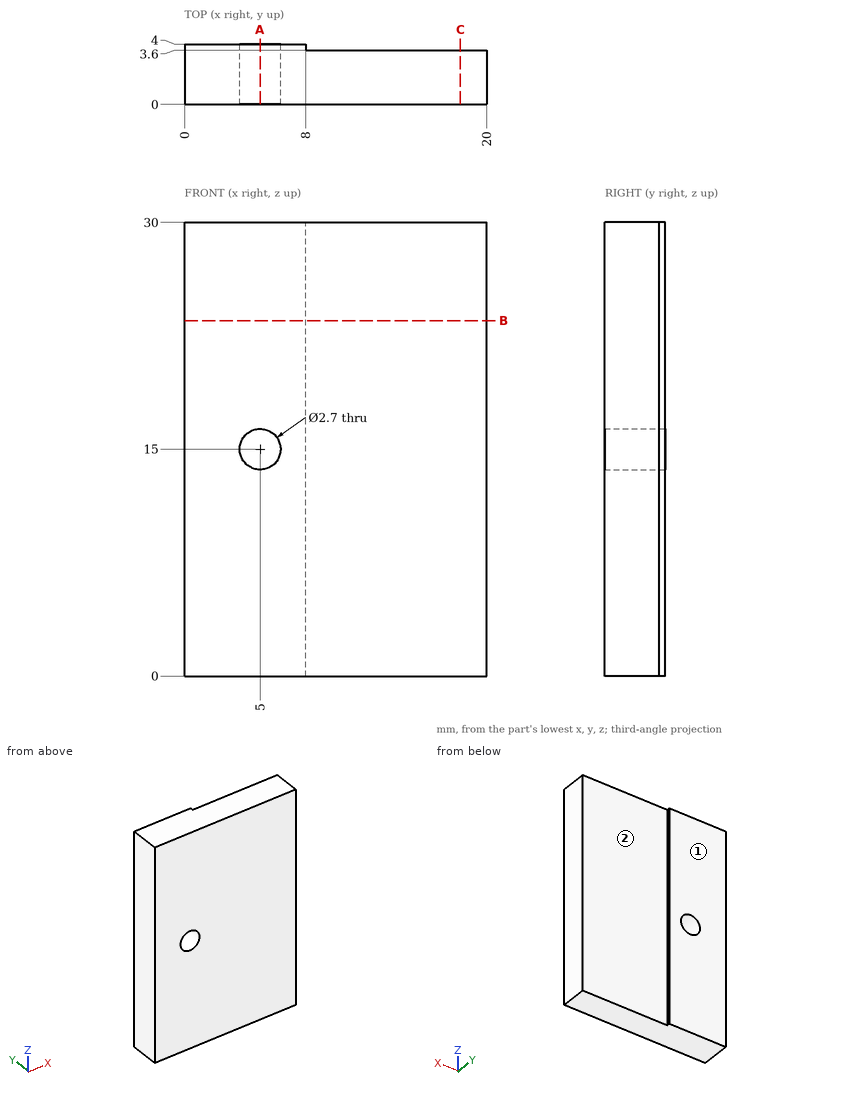
Here's the drawing with two shaded views (mm, measured from the low corner). I have some questions. A direction names the side the tool comes from. Coordinates: 2 decimals unless noted, no trailing zeros. Loops run counter-clockwise (first coordinate to the right, second up) from the corner with the lowest first, then second, coordinate; pieces in that order, holes last. Notation, with made-up numbers: M 76,41.5 L 80,41.5 A30 ccw 80,74.5 Z; hole C 26,30.5 d3. An arc over 180 degrees is marked long. Put each result on its own line as item: value. Start each with the question number.
(1) Will this pin go through, and if not, where does the flat tip stop? pin 1 Ø4 at (x, z) = (16.5, 16.5) entering from +Y.
(2) Imagine slicing it at C-C on x = 18.25. List the corners of the cut face in (y, z) for me.
(3) Which directions (+Z, -Z, +X, -X, +Y, -Y) give clear straight access to the entire face, cutting with the end or side of a thin tool? Please do the marked faces 1 and 2.
(4) Imagine slicing it at A-A on x = 5. List the corners of the cut face in (y, z) for me.
(5) I need wall thicknesses on probe 1 along Z at (x, y) = (5, 2.5); probe 2 along Y at (x, z) = (14, 20.5). Which ranges of each line are inside material? Lowest first, please.
(6) Imagine slicing it at B-B on z = 23.5. List the corners of the cut face in (x, y) for me, and give its area (3 significant figures).
Worked answers:
1. pin 1: stops at y = 3.6
2. outline: M 0,0 L 3.6,0 L 3.6,30 L 0,30 Z
3. face 1: +Z, -Z, +X, -X, +Y
3. face 2: +Z, -Z, +X, +Y
4. outline: M 0,0 L 4,0 L 4,13.65 L 0,13.65 Z; M 0,16.35 L 4,16.35 L 4,30 L 0,30 Z
5. probe 1: z = 0 to 13.65, 16.35 to 30
5. probe 2: y = 0 to 3.6
6. outline: M 0,0 L 20,0 L 20,3.6 L 8,3.6 L 8,4 L 0,4 Z
6. area: 75.2 mm2
